Read the model definition and answer for the solid it produces. Units are mm, in the model's axes. A direction names the side the tool comes from. Give positions to 0.01 mm unless a question says otherwise; leave off trailing zeros. Order: outer loops, then holes, each group sorted by start corner. A loop starts at its lowest first (then second) coordinate and runs counter-clockwise, first axis right, second up.
Item 1: A cutting plane is placed at A-A (x = -5). Write down the section's boundary in (y, z).
Item 2: Given pin 1 Ø6 at (y, z) = (27, 26) entering from -X; pin 2 Ø10 at (x, y) = (-12, 16) entering from +Z; pin 3 Ø1.6 at (x, y) = (-38, 27.5) entering from -Z, each flat-ended and moving along its own axis, determine where each tip first touches the part or whether it passes through.
Item 3: Which of the six approach directions +Z, -Z, +X, -X, +Y, -Y give full straight-line access (tool end or side, diameter ignored) to faces 1 (the face through (-38, 20, 20)), 2 (the face through (-10, 20, 36.8)), 3 (the face through (-20, 20, 10))?
Item 4: A cutting plane is placed at B-B (z = 6). Write down the section's boundary in (x, y), plus the area to 3 significant figures.
Item 5: Find the intervals of material crossed by line 1 along Z through (x, y) = (-18, 37); line 2 along X through (y, z) = (12, 14); line 3 along X through (y, z) = (21.5, 20.5), in increasing order.
from build123d import *

# Parameters (mm, degrees)
BOSS_EXTRUDE1_DEPTH = 40
FILLET1_SIZE        = 20


with BuildPart() as part:
    # Sketch2 → Boss-Extrude1 (new body)
    with BuildSketch(Plane(origin=(0, 0, 0), x_dir=(1, 0, 0), z_dir=(0, 1, 0))):
        Polygon((-20, -40), (-20, -36.8), (0, -36.8), (0, -20), (-20, -20), (-20, 0), (-36.8, 0), (-36.8, -20), (-40, -20), (-40, -40), align=None)
    extrude(amount=BOSS_EXTRUDE1_DEPTH)

    # Fillet1
    # a fillet whose section is not a circle: 20 mm, written as the material it takes off along each edge
    with BuildSketch(Plane(origin=(-40, -50, 40), x_dir=(0, 0, -1), z_dir=(0, 1, 0))) as fillet1_piece_1:
        with BuildLine():
            add(Edge.make_bspline([(FILLET1_SIZE, 0), (FILLET1_SIZE * 0.831801948466, 0), (FILLET1_SIZE * 0.663603896932, 0), (FILLET1_SIZE * 0.292893218813, -FILLET1_SIZE * 0.0716919198361), (FILLET1_SIZE * 0.0716919198361, -FILLET1_SIZE * 0.292893218813), (0, -FILLET1_SIZE * 0.663603896932), (0, -FILLET1_SIZE * 0.831801948466), (0, -FILLET1_SIZE)], knots=[0, 0, 0, 0, 0, 0, 0.5, 0.5, 1, 1, 1, 1, 1, 1], degree=5))
            Line((0, -FILLET1_SIZE), (0, 0))
            Line((0, 0), (FILLET1_SIZE, 0))
        make_face()
    extrude(amount=140, mode=Mode.SUBTRACT)


solid = part.part
Response values:
1. outline: (0, 20) - (40, 20) - (40, 36.8) - (0, 36.8) - close
2. pin 1: stops at x = -39.96
2. pin 2: stops at z = 36.8
2. pin 3: stops at z = 20
3. face 1: -Z, -X, +Y, -Y
3. face 2: +Z, +X, +Y, -Y
3. face 3: -Z, +X, +Y, -Y
4. outline: (-36.8, 0) - (-20, 0) - (-20, 40) - (-36.8, 40) - close
4. area: 672 mm2
5. line 1: z = 20 to 36.8
5. line 2: x = -36.8 to -20
5. line 3: x = -40 to 0
